Geometry: final body of the model. Coordinates: model frame, mm. Face numbers are marked on the shaded views. A direction names the side the tool comes from. Give positions to 0.01 mm unless a question says otherwise; leave off trailing zeros. Write each loop counter-clockwise with the first axis right and the second up, starting at its lowest first coordinate (ties: lowest second). Pieces come first, ordered by that corner, then holes.
```python
from build123d import *

# Parameters (mm, degrees)
SKETCH1_R                       = 9.525
SKETCH1_R_2                     = 3.175
BOSS_EXTRUDE1_DEPTH             = 95.25
SKETCH3_R                       = 12.7
SKETCH3_R_2                     = 9.525
BOSS_EXTRUDE2_DEPTH             = 3.175
SKETCH4_R                       = 6.35
BOSS_EXTRUDE3_DEPTH             = 19.05
TAP_DRILL_FOR_1_2_20_TAP1_D     = 11.50874
TAP_DRILL_FOR_1_2_20_TAP1_DEPTH = 19.05
CHAMFER1_SIZE                   = 1
CHAMFER1_SIZE2                  = 0.726542528
SKETCH8_W                       = 16.189039501
SKETCH8_H                       = 7.642767638
SKETCH8_H_2                     = 8.514884137
CUT_EXTRUDE1_DEPTH              = 6.35


with BuildPart() as part:
    # Sketch1 → Boss-Extrude1 (new body)
    with BuildSketch(Plane(origin=(0, 0, 0), x_dir=(1, 0, 0), z_dir=(0, 1, 0))):
        Circle(SKETCH1_R)
        Circle(SKETCH1_R_2, mode=Mode.SUBTRACT)
    extrude(amount=BOSS_EXTRUDE1_DEPTH)

    # Sketch3 → Boss-Extrude2 (add)
    with BuildSketch(Plane(origin=(0, 6.35, 0), x_dir=(-1, 0, 0), z_dir=(0, -1, 0))):
        Circle(SKETCH3_R)
        Circle(SKETCH3_R_2, mode=Mode.SUBTRACT)
    extrude(amount=-BOSS_EXTRUDE2_DEPTH)

    # Sketch4 → Boss-Extrude3 (add)
    with BuildSketch(Plane(origin=(0, 95.25, 0), x_dir=(1, 0, 0), z_dir=(0, 1, 0))):
        Circle(SKETCH4_R)
    extrude(amount=-BOSS_EXTRUDE3_DEPTH)

    # Tap Drill for 1/2-20 Tap1
    with Locations(Plane(origin=(0, 95.25, 0), x_dir=(1, 0, 0), z_dir=(0, 1, 0))):
        with Locations((0, 0)):
            Hole(TAP_DRILL_FOR_1_2_20_TAP1_D / 2, depth=TAP_DRILL_FOR_1_2_20_TAP1_DEPTH)

    # Chamfer1
    chamfer1_edges = [part.edges().sort_by_distance(p)[0] for p in [
        (-9.525, 9.525, 0),
    ]]
    chamfer1_side = [part.faces().sort_by_distance(p)[0] for p in [
        (12.340789755, 9.525, 0),
    ]]
    chamfer(chamfer1_edges, length=CHAMFER1_SIZE, length2=CHAMFER1_SIZE2, reference=chamfer1_side[0])

    # Sketch8 → Cut-Extrude1 (cut)
    with BuildSketch(Plane.XZ):
        with Locations((0.474519751, 10.171383819)):
            Rectangle(SKETCH8_W, SKETCH8_H)
        with Locations((0.474519751, -10.607442069)):
            Rectangle(SKETCH8_W, SKETCH8_H_2)
    extrude(amount=-CUT_EXTRUDE1_DEPTH, mode=Mode.SUBTRACT)


solid = part.part
```
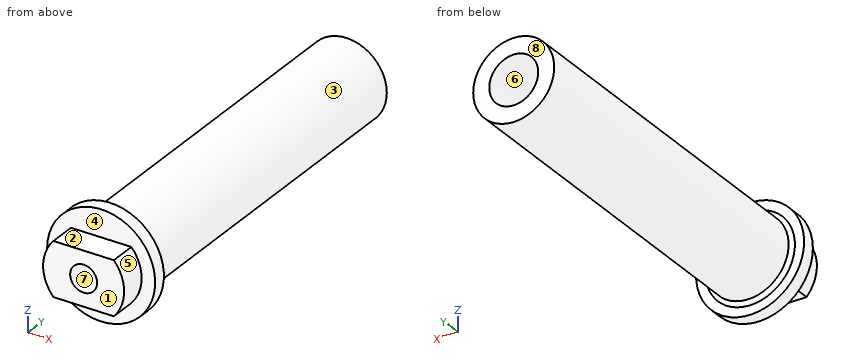
Item 1: Pull-direction query (X, two-part tool) for the marked faces 5, 6, 7 and 8; classes: +X half, -X half, draft (parallel to the pull), parting line (faces both ways), or undercut.
Found:
face 5: +X half
face 6: undercut
face 7: undercut
face 8: draft
Item 2: Section B-B, the plane z = 0. Return the cut outline in (x, y) (3 decimals), plus the area to 3 significant figures.
Found:
outline: (-12.7, 6.35) - (-9.525, 6.35) - (-9.525, 0) - (-3.175, 0) - (-3.175, 76.2) - (-5.754, 76.2) - (-5.754, 95.25) - (-9.525, 95.25) - (-9.525, 10.252) - (-10.525, 9.525) - (-12.7, 9.525) - close; (3.175, 0) - (9.525, 0) - (9.525, 6.35) - (12.7, 6.35) - (12.7, 9.525) - (10.525, 9.525) - (9.525, 10.252) - (9.525, 95.25) - (5.754, 95.25) - (5.754, 76.2) - (3.175, 76.2) - close
area: 1,130 mm2
Item 3: Section A-A, the plane x = 0. Return the cut outline in (y, z) (3 decimals).
Found:
outline: (0, -6.35) - (6.35, -6.35) - (6.35, -12.7) - (9.525, -12.7) - (9.525, -10.525) - (10.252, -9.525) - (95.25, -9.525) - (95.25, -5.754) - (76.2, -5.754) - (76.2, -3.175) - (0, -3.175) - close; (0, 3.175) - (76.2, 3.175) - (76.2, 5.754) - (95.25, 5.754) - (95.25, 9.525) - (10.252, 9.525) - (9.525, 10.525) - (9.525, 12.7) - (6.35, 12.7) - (6.35, 6.35) - (0, 6.35) - close
Item 4: Section C-C, the plane y = 44. Return the cut outline in (x, z) (3 decimals).
Found:
outline: circle Ø19.05 at (0, 0); hole circle Ø6.35 at (0, 0)
Item 5: Line query: L1, parallel to Z at x = 0, y = 44.5 (3 decimals); L2, parallel to Y at x = 9, z = 6 (3 decimals); L3, parallel to Z at x = 0, y = 87.75 (3 decimals). Output: solid intervals per line, ascending.
Found:
L1: z = -9.525 to -3.175, 3.175 to 9.525
L2: y = 6.35 to 9.525
L3: z = -9.525 to -5.754, 5.754 to 9.525
Item 6: Pin query (flat end, axial travel): pin 1 Ø8 at (y, z) = (64, 2) entering from +X (3 decimals); pin 2 Ø12 at (x, y) = (2, 18) entering from +Z (3 decimals); pin 3 Ø1 at (x, y) = (-5, 68) entering from +Z (3 decimals); pin 4 Ø5 at (x, z) = (7.5, 8.5) entering from +Y. Return the tip coordinate at first contact, or that it passes through.
Found:
pin 1: stops at x = 9.525
pin 2: stops at z = 9.525
pin 3: stops at z = 8.395
pin 4: stops at y = 95.25
Item 7: Reachability of the marked faces 1, 2, 3 and 4 from +Z, -Z, +X, -X, +Y, -Y: full face, straight path, thin tool, end or side. Return the list, or none.
Found:
face 1: +Z, -Z, +X, -X, -Y
face 2: +Z, +X, -X, -Y
face 3: +Y
face 4: -Y
